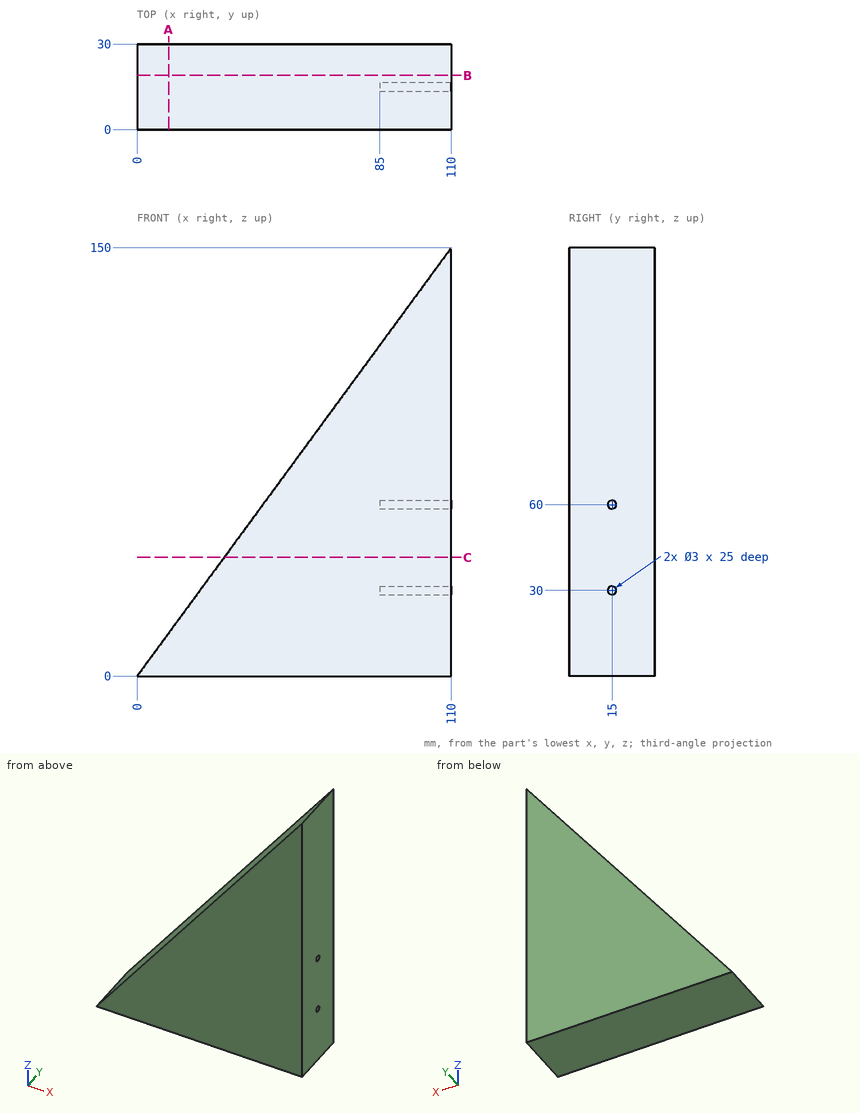
The figure shows three views and two pictorial views of one solid part (mm, origin at its lowest corner). Answer the questions. Coordinates: 2 decimals unless noted, no trailing zeros. Loops run counter-clockwise (first coordinate to the right, second up) from the corner with the lowest first, then second, coordinate; pieces in that order, holes last. Notation, with made-up numbers: (31.25, 20.5) -> (39.25, 20.5) arc R3 cw to (39.25, 25.5) -> close; hole circle Ø10 at (2.5, 58). An arc over 180 degrees is marked (long way). Return JSON: item names as keys, results as strings. Group by question number.
(1) A cutting plane is placed at C-C on z = 41.5. Write down the section's boundary in (x, y), and give its area (3 significant figures).
(2) Given pin 1 Ø3 at (x, y) = (43, 10) entering from +Z; pin 2 Ø3 at (x, y) = (28, 11.5) entering from +Z; pin 3 Ø6 at (y, z) = (12.5, 126.5) entering from -X, each flat-ended and moving along its own axis, determine where each tip first touches the part or whether it passes through.
(3) Find the intervals of material crossed by probe 1 along Z at (x, y) = (91.5, 15); probe 2 along Z at (x, y) = (94.5, 15); probe 3 along Z at (x, y) = (17, 4), in increasing order. Write a range as from..to.
(4) A cutting plane is placed at B-B on y = 19. Write down the section's boundary in (x, z).
(5) A cutting plane is placed at A-A on x = 11. Write down the section's boundary in (y, z), and give its area (3 significant figures).
The answers:
{
 "1": {"outline": "(30.43, 0) -> (110, 0) -> (110, 30) -> (30.43, 30) -> close", "area": "2,390 mm^2"},
 "2": {"pin 1": "stops at z = 60.68", "pin 2": "stops at z = 40.23", "pin 3": "stops at x = 90.57"},
 "3": {"probe 1": "z = 0..28.5, 31.5..58.5, 61.5..124.77", "probe 2": "z = 0..28.5, 31.5..58.5, 61.5..128.86", "probe 3": "z = 0..23.18"},
 "4": {"outline": "(0, 0) -> (110, 0) -> (110, 150) -> close"},
 "5": {"outline": "(0, 0) -> (30, 0) -> (30, 15) -> (0, 15) -> close", "area": "450 mm^2"}
}
